Autodesk Inventor part; units mm, degrees
ref_plane "YZ Plane" through (0, 0, 0) normal (1, 0, 0) x (0, 1, 0)
ref_plane "XZ Plane" through (0, 0, 0) normal (0, 1, 0) x (-1, 0, 0)
ref_plane "XY Plane" through (0, 0, 0) normal (0, 0, 1) x (1, 0, 0)
sketch "Sketch1" plane through (0, 0, 0) normal (0, 0, 1) x (1, 0, 0)
  line L0 (-25, 6.5) -> (0, 6.5)
  line L1 (0, 6.5) -> (0, -6.5)
  line L2 (0, -6.5) -> (-25, -6.5)
  line L3 (-25, -6.5) -> (-25, 6.5)
  point P0 (0, 0)
  point P1 (0, 0)
  dimension "d0" = 13
  dimension "d2" = 25
extrude "Extrusion1" add sketch "Sketch1" along normal blind 5
sketch "Sketch2" plane through (-25, -6.5, 0) normal (0, -1, 0) x (1, 0, 0)
  line L0 (25, 0) -> (25, 5)
  line L1 (0, 0) -> (60, 0)
  line L2 (60, 0) -> (60, 25)
  line L3 (60, 25) -> (0, 25)
  line L4 (0, 25) -> (0, 0)
  dimension "d5" = 35
  dimension "d6" = 25
extrude "Extrusion2" add sketch "Sketch2" against normal blind 2
fillet "Fillet1" radius 12.5 3 edges at (35, -5.5, 0) (35, -5.5, 25) (-25, -5.5, 25)
sketch "Sketch4" plane through (-25, -4.5, 0) normal (0, 1, 0) x (1, 0, 0)
  arc A0 (47.5, -25) -> (47.5, 0) centre (47.5, -12.5) ccw
  circle A1 centre (47.5, -12.5) radius 7.5
  dimension "d10" = 15
extrude "Extrusion3" add sketch "Sketch4" along normal blind 1
chamfer "Chamfer1" distance 1 angle 45 1 edges at (15, -4.5, 12.5)
sketch "Sketch5" plane through (22.5, -3.5, 12.5) normal (0, 1, 0) x (1, 0, 0)
  circle A0 centre (0, 0) radius 7.5
  circle A1 centre (0, 0) radius 3.75
  point P0 (-22.5, 12.5)
  dimension "d17" = 7.5
extrude "Extrusion4" add sketch "Sketch5" along normal blind 1.5 contours A1
sketch "Sketch6" plane through (0, 6.5, 5) normal (1, 0, 0) x (0, 0, -1)
  line L0 (-3.75, -8.5) -> (-11.25, -8.5)
  line L1 (-11.25, -10) -> (-3.75, -10)
  line L2 (-3.75, -10) -> (-5.25, -8.5)
  line L3 (-3.75, -8.5) -> (-3.75, -10)
  line L4 (-3.75, -8.5) -> (-5.25, -8.5)
  point P0 (5, -6.5)
extrude "Extrusion5" cut sketch "Sketch6" along normal through all
mirror "Mirror1" about plane through (0, 0, 0) normal (0, 1, 0) of "Extrusion4", "Extrusion3", "Chamfer1", "Fillet1", "Extrusion2", "Extrusion5"
sketch "Sketch7" plane through (0, 0, 5) normal (0, 0, 1) x (1, 0, 0)
  line L0 (-25, 4.5) -> (-25, -4.5)
  line L1 (0, -4.5) -> (0, 4.5)
  line L2 (-25, 0) -> (0, 0)
  circle A0 centre (-20, 0) radius 1.55
  circle A1 centre (-5, 0) radius 1.55
  dimension "d23" = 5
  dimension "d24" = 5
  dimension "d25" = 3.1
extrude "Extrusion6" cut sketch "Sketch7" against normal through all
sketch "Sketch8" plane through (0, 0, 5) normal (0, 0, 1) x (1, 0, 0)
  circle A0 centre (-5, 0) radius 1.55
  circle A1 centre (-20, 0) radius 1.55
  line L0 (-16.7668, 0) -> (-18.3834, -2.8)
  line L1 (-18.3834, -2.8) -> (-21.6166, -2.8)
  line L2 (-21.6166, -2.8) -> (-23.2332, 0)
  line L3 (-23.2332, 0) -> (-21.6166, 2.8)
  line L4 (-21.6166, 2.8) -> (-18.3834, 2.8)
  line L5 (-18.3834, 2.8) -> (-16.7668, 0)
  line L6 (-8.2332, 0) -> (-6.6166, 2.8)
  line L7 (-6.6166, 2.8) -> (-3.3834, 2.8)
  line L8 (-3.3834, 2.8) -> (-1.7668, 0)
  line L9 (-1.7668, 0) -> (-3.3834, -2.8)
  line L10 (-3.3834, -2.8) -> (-6.6166, -2.8)
  line L11 (-6.6166, -2.8) -> (-8.2332, 0)
  point P0 (0, 0)
  dimension "d28" = 5.6
extrude "Extrusion7" cut sketch "Sketch8" against normal blind 2.5
sketch "Sketch9" plane through (-12.5, 6.5, 25) normal (0, 1, 0) x (1, 0, 0)
  arc A0 (35, 0) -> (35, 25) centre (35, 12.5) ccw
  circle A1 centre (35, 12.5) radius 1.6
  point P0 (12.5, 25)
  dimension "d32" = 3.2
extrude "Extrusion8" cut sketch "Sketch9" against normal through all
sketch "Sketch10" plane through (-12.5, 6.5, 25) normal (0, 1, 0) x (1, 0, 0)
  circle A0 centre (35, 12.5) radius 1.6
  arc A1 (35, 0) -> (35, 25) centre (35, 12.5) ccw
  circle A2 centre (35, 12.5) radius 3.25
  point P0 (12.5, 25)
  dimension "d36" = 6.5
extrude "Extrusion9" cut sketch "Sketch10" against normal blind 3
sketch "Sketch11" plane through (-12.5, -6.5, 25) normal (0, -1, 0) x (1, 0, 0)
  circle A0 centre (35, -12.5) radius 1.6
  arc A1 (35, -25) -> (35, 0) centre (35, -12.5) ccw
  line L0 (31.7668, -12.5) -> (33.3834, -9.7)
  line L1 (33.3834, -9.7) -> (36.6166, -9.7)
  line L2 (36.6166, -9.7) -> (38.2332, -12.5)
  line L3 (38.2332, -12.5) -> (36.6166, -15.3)
  line L4 (36.6166, -15.3) -> (33.3834, -15.3)
  line L5 (33.3834, -15.3) -> (31.7668, -12.5)
  point P0 (12.5, -25)
  point P1 (35, -9.7)
  dimension "d40" = 5.6
extrude "Extrusion10" cut sketch "Sketch11" against normal blind 3
properties part number "z pulley holder"
Input: part model. Units: mm. Frame: model coordinates. A direction names the side the tool comes from. Give positions to 0.01 mm unless a question says otherwise; leave off trailing zeros. Loops run counter-clockwise (first coordinate to the right, second up) from the corner with the lowest first, then second, coordinate; pieces in that order, holes last. Notation, with made-up numbers: M 53.25,27.25 L 96.25,27.25 A23 cw 96.25,48.25 Z; hole C -7,-17.5 d7. An arc over 180 degrees is marked long. Answer as CSV lines item,"result". Start each with the question number.
1. Reachability of faces 4 (the face through (-5, -2.8, 4)), 5 (the face through (20.086, -5.021, 11.08)), 6 (the face through (20.62, -3.5, 9.06)) from +Z, -Z, +X, -X, +Y, -Y: full face, straight path, thin tool, end or side. Return the list, or none.
2. Section A-A on x = -5. Return loops of the section in (y, z).
3. Pin query (flat end, axial travel): P1, Ø4.5, axis at x = -19, y = -0.5, coming from the +Z side; P2, Ø6, axis at x = 22.5, z = 12.5, coming from the +Y side; P3, Ø4, axis at y = 1, z = 3, coming from the +X side. Return the tip coordinate at first contact, or that it passes through.
4. Section C-C on x = -15. Return loops of the section in (y, z), plus the area to 3 significant figures.
5. Pull-direction query (X, two-part tool) for faces 1 (the face through (-21.241, 5.486, 21.436)), 2 (the face through (-2.564, -1.38, 3.768)), 3 (the face through (-13, 0, 5)); classes: released by +X, released by -X, zero draft, split by the parting line, or undercut.
6. Line query: L1, parallel to Y at x = 28.5, z = 20.75; L2, parallel to Y at x = -20, z = 1.45; L3, parallel to Z at x = 22.5, y = 4.6. Output: solid intervals per line, ascending.
7. Section B-B on z = 22. Return loops of the section in (x, y), plus the area to 3 significant figures.
8. Section D-D on x = 23.5. State how many separate pieces and enclosed holes the cut face has, plus the area to 3 significant figures.
Computed values:
1,face 4,"+Z"
1,face 5,"-Y"
1,face 6,"none"
2,outline,"M -6.5,0 L -1.55,0 L -1.55,2.5 L -2.8,2.5 L -2.8,5 L -4.5,5 L -4.5,25 L -6.5,25 Z; M 1.55,0 L 6.5,0 L 6.5,25 L 4.5,25 L 4.5,5 L 2.8,5 L 2.8,2.5 L 1.55,2.5 Z"
3,P1,"stops at z = 5"
3,P2,"stops at y = 3.5"
3,P3,"stops at x = 0"
4,outline,"M -6.5,0 L 6.5,0 L 6.5,24.75 L 4.5,24.75 L 4.5,5 L -4.5,5 L -4.5,24.75 L -6.5,24.75 Z"
4,area,"144 mm²"
5,face 1,"released by -X"
5,face 2,"undercut"
5,face 3,"zero draft"
6,L1,"y = -6.5 to -4.5, 4.5 to 6.5"
6,L2,"y = -6.5 to -1.55, 1.55 to 6.5"
6,L3,"z = 0 to 9.25, 15.75 to 25"
7,outline,"M -20.62,-6.5 L 30.62,-6.5 L 30.62,-4.5 L -20.62,-4.5 Z; M -20.62,4.5 L 30.62,4.5 L 30.62,6.5 L -20.62,6.5 Z"
7,area,"205 mm²"
8,separate pieces,"4"
8,enclosed holes,"0"
8,area,"108 mm²"
